```python
from build123d import *

# Parameters (mm, degrees)
SKETCH_2_W               = 42.3
SKETCH_2_H               = 42.3
EXTRUDE_2_DEPTH          = 8
CHAMFER_1_SIZE           = 3
SKETCH_3_W               = 42.3
SKETCH_3_H               = 42.3
EXTRUDE_3_DEPTH          = 22
EXTRUDE_4_DEPTH          = 8
CUT_EXTRUDE_1_DEPTH      = 22
CUT_EXTRUDE_START        = -8
CUT_EXTRUDE_4_DEPTH      = 22
SKETCH_7_R               = 11
EXTRUDE_5_DEPTH          = 1
SKETCH_8_R               = 2.5
EXTRUDE_6_DEPTH          = 22
CUT_EXTRUDE_6_DEPTH      = 18
HOLE_WIZARD_M3_1_D       = 2.5
SKETCH_15_W              = 42.295221422
SKETCH_15_H              = 22.0000003
CUT_EXTRUDE_8_DEPTH      = 0.5
PATTERN_CIRCULAR_1_COUNT = 4
CHAMFER_3_SIZE           = 0.1


with BuildPart() as part:
    # 草图2 → 凸台-拉伸2 (new body)
    with BuildSketch(Plane(origin=(0, 0, 0), x_dir=(1, 0, 0), z_dir=(0, 1, 0))):
        Rectangle(SKETCH_2_W, SKETCH_2_H)
    extrude(amount=EXTRUDE_2_DEPTH)

    # 倒角1
    chamfer_1_edges = [part.edges().sort_by_distance(p)[0] for p in [
        (21.15, 4, 21.15),
        (-21.15, 4, 21.15),
        (-21.15, 4, -21.15),
        (21.15, 4, -21.15),
    ]]
    chamfer(chamfer_1_edges, length=CHAMFER_1_SIZE)

    # 草图3 → 凸台-拉伸3 (add)
    with BuildSketch(Plane(origin=(0, 8, 0), x_dir=(1, 0, 0), z_dir=(0, 1, 0))):
        Rectangle(SKETCH_3_W, SKETCH_3_H)
    extrude(amount=EXTRUDE_3_DEPTH)

    # 草图4 → 凸台-拉伸4 (add)
    with BuildSketch(Plane(origin=(0, 30, 0), x_dir=(1, 0, 0), z_dir=(0, 1, 0))):
        Polygon((-21.15, 18.15), (-21.15, -18.15), (-18.15, -21.15), (18.15, -21.15), (21.15, -18.15), (21.15, 18.15), (18.15, 21.15), (-18.15, 21.15), align=None)
    extrude(amount=EXTRUDE_4_DEPTH)

    # 草图5 → 切除-拉伸1 (cut)
    with BuildSketch(Plane(origin=(0, 30, 0), x_dir=(1, 0, 0), z_dir=(0, 1, 0))):
        Polygon((-16.15, 21.15), (-21.15, 21.15), (-21.15, 16.15), align=None)
    extrude(amount=-CUT_EXTRUDE_1_DEPTH, mode=Mode.SUBTRACT)

    # 草图6 → 切除-拉伸4 (cut)
    with BuildSketch(Plane(origin=(0, 38, 0), x_dir=(1, 0, 0), z_dir=(0, 1, 0)).offset(CUT_EXTRUDE_START)):
        Polygon((-16.15, -21.15), (-21.15, -16.15), (-21.15, -18.15), (-18.15, -21.15), align=None)
        Polygon((-18.15, -21.15), (-21.15, -18.15), (-21.15, -21.15), align=None)
        Polygon((21.15, -16.15), (16.15, -21.15), (18.15, -21.15), (21.15, -18.15), align=None)
        Polygon((21.15, -18.15), (18.15, -21.15), (21.15, -21.15), align=None)
        Polygon((18.15, 21.15), (16.15, 21.15), (21.15, 16.15), (21.15, 18.15), align=None)
        Polygon((21.15, 21.15), (18.15, 21.15), (21.15, 18.15), align=None)
    extrude(amount=-CUT_EXTRUDE_4_DEPTH, mode=Mode.SUBTRACT)

    # 草图7 → 凸台-拉伸5 (add)
    with BuildSketch(Plane(origin=(0, 38, 0), x_dir=(1, 0, 0), z_dir=(0, 1, 0))):
        with Locations(Location((0, 0, 0), (0, 0, 270))):
            Circle(SKETCH_7_R)
    extrude(amount=EXTRUDE_5_DEPTH)

    # 草图8 → 凸台-拉伸6 (add)
    with BuildSketch(Plane(origin=(0, 39, 0), x_dir=(1, 0, 0), z_dir=(0, 1, 0))):
        with Locations(Location((0, 0, 0), (0, 0, 270))):
            Circle(SKETCH_8_R)
    extrude(amount=EXTRUDE_6_DEPTH)

    # 草图9 → 切除-拉伸6 (cut)
    with BuildSketch(Plane(origin=(0, 61, 0), x_dir=(1, 0, 0), z_dir=(0, 1, 0))):
        Polygon((-76.274840795, 2), (-1.5, 2), (1.5, 2), (76.274840795, 2), (76.274840795, 151.54968159), (-76.274840795, 151.54968159), align=None)
    extrude(amount=-CUT_EXTRUDE_6_DEPTH, mode=Mode.SUBTRACT)

    # M3 螺纹孔1 (through all)
    with Locations(Plane(origin=(0, 38, 0), x_dir=(1, 0, 0), z_dir=(0, 1, 0))):
        with Locations((-15.5, 15.5), (15.5, 15.5), (15.5, -15.5), (-15.5, -15.5)):
            Hole(HOLE_WIZARD_M3_1_D / 2)

    # 草图15 → 切除-拉伸8 (cut)
    with BuildSketch(Plane.ZY.offset(21.15)):
        with Locations((-0.002389289, 18.99999985)):
            Rectangle(SKETCH_15_W, SKETCH_15_H)
    cut_extrude_8 = extrude(amount=-CUT_EXTRUDE_8_DEPTH, mode=Mode.SUBTRACT)

    # 阵列(圆周)1: 切除-拉伸8 ×4 about axis
    pattern_circular_1_axis = Axis((0, 0, 0), (0, 1, 0))
    for i in range(1, PATTERN_CIRCULAR_1_COUNT):
        add(cut_extrude_8.rotate(pattern_circular_1_axis, i * 360 / PATTERN_CIRCULAR_1_COUNT), mode=Mode.SUBTRACT)

    # 倒角3
    chamfer_3_edges = [part.edges().sort_by_distance(p)[0] for p in [
        (2.371708245, 61, 0.790569415),
    ]]
    chamfer(chamfer_3_edges, length=CHAMFER_3_SIZE)


solid = part.part
```
Check sheet for the modelled part. Datum: model origin and axes. Units: mm. A direction names the side the tool comes from. Coordinates: 2 decimals unless noted, no trailing zeros. Order: outer loops, then holes, each group sorted by start corner. A loop starts at its lowest first (then second) coordinate and runs counter-clockwise, first axis right, second up. Notation, with made-up numbers: M 29.25,46.25 L 58.25,46.25 A15 ccw 58.25,63.25 Z; hole C 19,-25.75 d8. An arc over 180 degrees is marked long. One line per question, with ' | ' between items. Start each with the question number.
Item 1: Sectioned sample at A-A on z = -15.5. Record the cut outline in (x, y), and give its area (3 significant figures).
Item 2: Sectioned sample at B-B on x = 15.5. Record the cut outline in (y, z), and give its area (3 significant figures).
Item 3: Access from +Z, -Z, +X, -X, +Y, -Y to the whole of each face (thin tool, end or side, straight path). Record for faces 1 (the cylindrical face through (0.751, 49.797, 2.385)), 2 (the flat face through (0, 19, 20.65)), 3 (the flat face through (-18.6, 19.2, 18.7)), 4 (the flat face through (19, 30, 19)), 5 (the flat face through (-20.65, 19, 0)).
Item 4: Sectioned sample at C-C on z = 0. Record the cut outline in (x, y).
Item 5: Gauge pin test, flat ends, axial feed: P1, Ø3, axis at x = -18.5, z = -18.5, coming from the +Y side; P2, Ø12, axis at x = -10, z = -9.5, coming from the +Y side; P3, Ø6, axis at x = 4, y = 52.5, coming from the +Z side. Record the tip position at first contact, or that the pin passes through.
Item 6: Mould release check, pull along Z, two halves, no side actions. Record for faces 6 (the flat face through (20.65, 19, 0)), 7 (the cylindrical face through (-14.579, 18.734, -16.345)), 8 (the flat face through (0, 4, 21.15)), 9 (the cylindrical face through (-15.34, 18.73, 14.26)): pulls with the +Z half, pulls with the -Z half, needs draft (parallel to the pull), parting line crosses it, or undercut.
Item 7: Sectioned sample at D-D on x = 0. Record the cut outline in (y, z).
Item 8: Material ranges on line 1 (X direction, y = 14.5, z = 15.5), recorded low to high.
Answer below:
1) outline: M -21.15,0 L -16.75,0 L -16.75,38 L -21.15,38 L -21.15,30 L -20.65,30 L -20.65,8 L -21.15,8 Z; M -14.25,0 L 14.25,0 L 14.25,38 L -14.25,38 Z; M 16.75,0 L 21.15,0 L 21.15,8 L 20.65,8 L 20.65,30 L 21.15,30 L 21.15,38 L 16.75,38 Z | area: 1,400 mm^2
2) outline: M 0,-21.15 L 8,-21.15 L 8,-20.65 L 30,-20.65 L 30,-21.15 L 38,-21.15 L 38,-16.75 L 0,-16.75 Z; M 0,-14.25 L 38,-14.25 L 38,14.25 L 0,14.25 Z; M 0,16.75 L 38,16.75 L 38,21.15 L 30,21.15 L 30,20.65 L 8,20.65 L 8,21.15 L 0,21.15 Z | area: 1,400 mm^2
3) face 1: +Y | face 2: +Z, +X, -X | face 3: +Z, -X | face 4: none | face 5: +Z, -Z, -X
4) outline: M -21.15,0 L 21.15,0 L 21.15,8 L 20.65,8 L 20.65,30 L 21.15,30 L 21.15,38 L 11,38 L 11,39 L 2.5,39 L 2.5,60.9 L 2.4,61 L -2.4,61 L -2.5,60.9 L -2.5,39 L -11,39 L -11,38 L -21.15,38 L -21.15,30 L -20.65,30 L -20.65,8 L -21.15,8 Z
5) P1: stops at y = 38 | P2: stops at y = 39 | P3: stops at z = 2.29
6) face 6: needs draft | face 7: undercut | face 8: pulls with the +Z half | face 9: undercut
7) outline: M 0,-21.15 L 8,-21.15 L 8,-20.65 L 30,-20.65 L 30,-21.15 L 38,-21.15 L 38,-11 L 39,-11 L 39,-2.5 L 43,-2.5 L 43,-2 L 61,-2 L 61,2.4 L 60.9,2.5 L 39,2.5 L 39,11 L 38,11 L 38,21.15 L 30,21.15 L 30,20.65 L 8,20.65 L 8,21.15 L 0,21.15 Z
8) line 1: x = -20.65 to -16.75, -14.25 to 14.25, 16.75 to 20.65
